```python
from build123d import *

# Parameters (mm, degrees)
BOSS_EXTRUDE1_DEPTH = 3
CHAMFER1_SIZE       = 1
FILLET1_R           = 1.25


with BuildPart() as part:
    # Sketch1 → Boss-Extrude1 (new body)
    with BuildSketch(Plane.XY):
        with BuildLine():
            ThreePointArc((4.563792029, -5.438915546), (0, 7.1), (-4.563792029, -5.438915546))
            ThreePointArc((-4.563792029, -5.438915546), (-4.329604045, -8.115696446), (-7.006384946, -8.34988443))
            ThreePointArc((-7.006384946, -8.34988443), (0, 10.9), (7.006384946, -8.34988443))
            ThreePointArc((7.006384946, -8.34988443), (4.329604045, -8.115696446), (4.563792029, -5.438915546))
        make_face()
    extrude(amount=BOSS_EXTRUDE1_DEPTH)

    # Chamfer1
    chamfer1_edges = [part.edges().sort_by_distance(p)[0] for p in [
        (0, 10.9, 0),
        (4.329604045, -8.115696446, 0),
        (0, 7.1, 0),
        (-4.329604045, -8.115696446, 0),
    ]]
    chamfer(chamfer1_edges, length=CHAMFER1_SIZE)

    # Fillet1
    fillet1_edges = [part.edges().sort_by_distance(p)[0] for p in [
        (4.329604045, -8.115696446, 3),
        (0, 10.9, 3),
        (-4.329604045, -8.115696446, 3),
        (0, 7.1, 3),
    ]]
    fillet(fillet1_edges, radius=FILLET1_R)


solid = part.part
```
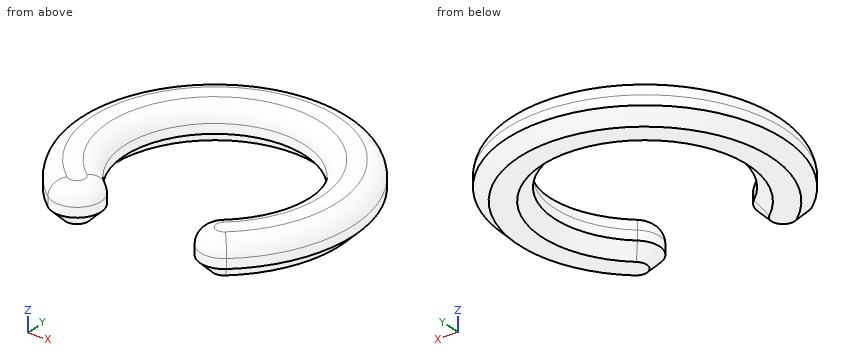
CAD build for the part. Positions are in the model's coordinates, mm. Round coordinates to 2 decimals unless told otherwise and drop trailing zeros. Write each loop counter-clockwise with the first axis right and the second up, starting at its lowest first coordinate (ties: lowest second). Pieces come first, ordered by that corner, then holes.
Item 1: Drill centre lines: L1, parallel to X at y = 0, z = 1.65; L2, parallel to Y at x = 0, z = 1.5; L3, parallel to X at y = 5.75, z = 1.45. Where is each one in solid material? Low to high.
Filled in:
L1: x = -10.9 to -7.1, 7.1 to 10.9
L2: y = 7.1 to 10.9
L3: x = -9.26 to -4.17, 4.17 to 9.26
Item 2: Band-saw the part on C-C on z = 1.5. Write the cut outline in (x, y).
Filled in:
outline: (-7.01, -8.35) arc R1.9 ccw to (-4.56, -5.44) arc R7.1 cw (long way) to (4.56, -5.44) arc R1.9 ccw to (7.01, -8.35) arc R10.9 ccw (long way) to start
Item 3: Band-saw the part on B-B on z = 0.3. Write the cut outline in (x, y), then the cut area to 3 significant figures.
Filled in:
outline: (-6.56, -7.81) arc R1.2 ccw to (-5.01, -5.98) arc R7.8 cw (long way) to (5.01, -5.98) arc R1.2 ccw to (6.56, -7.81) arc R10.2 ccw (long way) to start
area: 110 mm2
Item 4: Drop flat-ended pins along their axis: pin 1 Ø1.5 at (y, z) = (-2.5, 1) entering from +X; pin 2 Ø1 at (x, z) = (6.5, 2.5) entering from -Y; pin 3 Ø5 at (x, y) = (-8, 2) entering from -Z; pin 4 Ø1.5 at (x, y) = (3, 5) entering from -Z. Give the stop position or say it passes through.
Filled in:
pin 1: stops at x = 10.76
pin 2: stops at y = -8.7
pin 3: stops at z = 0
pin 4: passes through
Item 5: Band-saw the part on A-A on x = 0. Write the cut outline in (y, z).
Filled in:
outline: (7.1, 1) - (8.1, 0) - (9.9, 0) - (10.9, 1) - (10.9, 1.75) arc R1.25 ccw to (9.65, 3) - (8.35, 3) arc R1.25 ccw to (7.1, 1.75) - close
